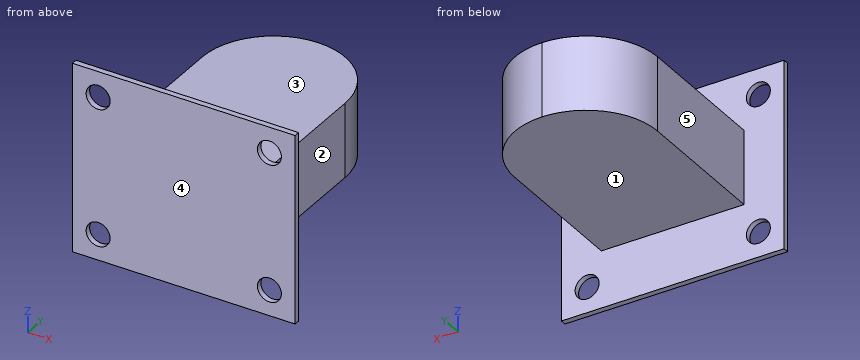
from build123d import *

# Parameters (mm, degrees)
SKETCH_1_W      = 39
SKETCH_1_H      = 33
SKETCH_1_R      = 2.1
EXTRUDE_1_DEPTH = 1
SKETCH_2_W      = 25
SKETCH_2_H      = 37
EXTRUDE_2_DEPTH = 6.5
FILLET_1_R      = 12.5


with BuildPart() as part:
    # 草图1 → 凸台-拉伸1 (new body)
    with BuildSketch(Plane(origin=(0, 0, 0), x_dir=(1, 0, 0), z_dir=(0, 1, 0))):
        Rectangle(SKETCH_1_W, SKETCH_1_H)
        with Locations(Location((-15, 12, 0), (0, 0, 270))):
            Circle(SKETCH_1_R, mode=Mode.SUBTRACT)
        with Locations(Location((15, 12, 0), (0, 0, 90))):
            Circle(SKETCH_1_R, mode=Mode.SUBTRACT)
        with Locations(Location((15, -12, 0), (0, 0, 270))):
            Circle(SKETCH_1_R, mode=Mode.SUBTRACT)
        with Locations(Location((-15, -12, 0), (0, 0, 90))):
            Circle(SKETCH_1_R, mode=Mode.SUBTRACT)
    extrude(amount=EXTRUDE_1_DEPTH)

    # 草图2 → 凸台-拉伸2 (add, symmetric)
    with BuildSketch(Plane.XY):
        with Locations((0, 19.5)):
            Rectangle(SKETCH_2_W, SKETCH_2_H)
    extrude(amount=EXTRUDE_2_DEPTH, both=True)

    # 圆角1
    fillet_1_edges = [part.edges().sort_by_distance(p)[0] for p in [
        (-12.5, 38, 0),
        (12.5, 38, 0),
    ]]
    fillet(fillet_1_edges, radius=FILLET_1_R - 0.0001)  # a hair under: the kernel refuses the full size


solid = part.part
Design review of the part built by this model. Coordinates are the model's own, in mm. Face numbers are marked on the shaded views. A direction names the side the tool comes from. Round coordinates to 2 decimals unless told otherwise and drop trailing zeros. Write each loop counter-clockwise with the first axis right and the second up, starting at its lowest first coordinate (ties: lowest second). Pieces come first, ordered by that corner, then holes. Notation, with made-up numbers: (-30.75, -32.75) - (5.25, -32.75) arc R19 cw to (5.25, -27.75) - close; hole circle Ø9 at (86, 51.25). An arc over 180 degrees is marked (long way). Return JSON: item names as keys, results as strings. Group by question number.
Item 1: Machinability: for the marked faces 1, 2, 3, 4 and 5, which of the approach directions +Z, -Z, +X, -X, +Y, -Y give a long, thin tool a straight path to every point of the face, cutting with its end or side? Answer none if there is none.
Item 2: We need section A-A on x = -15. Write out the cut boundary in (y, z), and give its area (3 significant figures).
Item 3: We need section B-B on z = -12. Write out the cut boundary in (x, y).
Item 4: We need section D-D on y = 3. Write out the cut boundary in (x, z).
Item 5: Insertion check: P1, Ø10.5, axis at y = 11.5, z = -1, coming from the -X side; P2, Ø1, axis at x = -7.5, y = 10, coming from the +Z side; P3, Ø14.5, axis at y = 9, z = -2, coming from the +X side. Each pin has a flat end and moves straight along its axis. Give the tip position at first contact, or say it passes through.
Item 6: For probe 1 along X at (y, z) = (0.35, 12); probe 2 along Y at (x, z) = (14, 7); probe 3 along Z at (x, y) = (-6.5, 12.5), list the stretches that pass through material, from the lowest coordinate up. Write a range as [from, to].
Model answer:
{
 "1": {"face 1": "-Z, +X, -X, +Y", "face 2": "+Z, -Z, +X, +Y", "face 3": "+Z, +X, -X, +Y", "face 4": "+Z, -Z, +X, -X, -Y", "face 5": "+Z, -Z, -X, +Y"},
 "2": {"outline": "(0, -16.5) - (1, -16.5) - (1, -14.1) - (0, -14.1) - close; (0, -9.9) - (1, -9.9) - (1, 9.9) - (0, 9.9) - close; (0, 14.1) - (1, 14.1) - (1, 16.5) - (0, 16.5) - close", "area": "24.6 mm²"},
 "3": {"outline": "(-19.5, 0) - (-17.1, 0) - (-17.1, 1) - (-19.5, 1) - close; (-12.9, 0) - (12.9, 0) - (12.9, 1) - (-12.9, 1) - close; (17.1, 0) - (19.5, 0) - (19.5, 1) - (17.1, 1) - close"},
 "4": {"outline": "(-12.5, -6.5) - (12.5, -6.5) - (12.5, 6.5) - (-12.5, 6.5) - close"},
 "5": {"P1": "stops at x = -12.5", "P2": "stops at z = 6.5", "P3": "stops at x = 12.5"},
 "6": {"probe 1": "x = [-19.5, -17.1], [-12.9, 12.9], [17.1, 19.5]", "probe 2": "y = [0, 1]", "probe 3": "z = [-6.5, 6.5]"}
}
